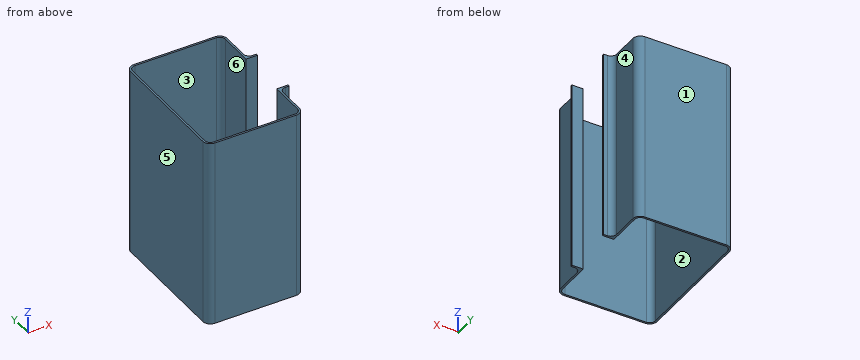
```python
from build123d import *

# Parameters (mm, degrees)
F1_DEPTH = 100


# Not quite as in the source:
# - a feature names something its author has since deleted; it is built from what else it names


with BuildPart() as f1:
    # F0 (on Top) → F1 (new body)
    with BuildSketch(Plane.XY):
        with BuildLine():
            Line((-21.5, 35), (21.5, 35))
            ThreePointArc((21.5, 35), (23.6213203436, 34.1213203436), (24.5, 32))
            Line((24.5, 32), (24.5, 13.625))
            Line((24.5, 13.625), (30.5, 13.625))
            Line((30.5, 13.625), (30.5, 14.625))
            Line((30.5, 14.625), (28.5, 14.625))
            ThreePointArc((28.5, 14.625), (26.3786796564, 15.5036796564), (25.5, 17.625))
            Line((25.5, 17.625), (25.5, 32))
            ThreePointArc((25.5, 32), (24.3284271247, 34.8284271247), (21.5, 36))
            Line((21.5, 36), (-21.5, 36))
            ThreePointArc((-21.5, 36), (-24.3284271247, 34.8284271247), (-25.5, 32))
            Line((-25.5, 32), (-25.5, -32))
            ThreePointArc((-25.5, -32), (-24.3284271247, -34.8284271247), (-21.5, -36))
            Line((-21.5, -36), (21.5, -36))
            ThreePointArc((21.5, -36), (24.3284271247, -34.8284271247), (25.5, -32))
            Line((25.5, -32), (25.5, -17.625))
            ThreePointArc((25.5, -17.625), (26.3786796564, -15.5036796564), (28.5, -14.625))
            Line((28.5, -14.625), (30.5, -14.625))
            Line((30.5, -14.625), (30.5, -13.625))
            Line((30.5, -13.625), (24.5, -13.625))
            Line((24.5, -13.625), (24.5, -32))
            ThreePointArc((24.5, -32), (23.6213203436, -34.1213203436), (21.5, -35))
            Line((21.5, -35), (-21.5, -35))
            ThreePointArc((-21.5, -35), (-23.6213203436, -34.1213203436), (-24.5, -32))
            Line((-24.5, -32), (-24.5, 32))
            ThreePointArc((-24.5, 32), (-23.6213203436, 34.1213203436), (-21.5, 35))
        make_face()
    extrude(amount=F1_DEPTH)


solid = f1.part
```
Geometry: final body of the model. Coordinates: model frame, mm. Face numbers are marked on the shaded views. A direction names the side the tool comes from. Round coordinates to 2 decimals unless told otherwise and drop trailing zeros. Write each loop counter-clockwise with the first axis right and the second up, starting at its lowest first coordinate (ties: lowest second). Pieces come first, ordered by that corner, then holes. Notation, with made-up numbers: M 22.25,-1.75 L 50.25,-1.75 A14 ccw 50.25,7.25 Z; hole C -17,57 d9. An arc over 180 degrees is marked long. Answer in a Markdown table with one row per item. Add a question column.
(1) Draft query along X for the marked faces 1, 2, 3 and 4. Return one class per face: pulls with the +X half, pulls with the -X half, needs draft (parallel to the pull), parting line crosses it, or undercut.
(2) Contact query for flat-ended pins moving along their axis: pin 1 (4.5 mm diameter, centred on y = 26, z = 57.5, fed in from +X); pin 2 (1.5 mm diameter, centred on y = 0.5, z = 78.5, fed in from +X); pin 3 (3 mm diameter, centred on x = 28.5, z = 53, fed in from +Y). Output: stop coordinate, or through.
(3) Cut plane B-B, the plane x = -16.5. Return the cut outline in (y, z), then the cut area to 3 significant figures.
(4) Ray query, L1, parallel to Y at x = 11, z = 9; L2, parallel to X at y = 21.5, z = 56; L3, parallel to X at y = 3.5, z = 18. Return the intervals inside material, ascending.
(5) Cut plane C-C, the plane z = 36. Return the cut outline in (x, y) (3 decimals), then the cut area to 3 significant figures.
(6) Cut plane D-D, the plane y = 0.5. Return the cut outline in (x, z), then the cut area to 3 significant figures.
(7) Cut plane A-A, the plane y = -23. Return the cut outline in (x, z).
(8) Reachability of the marked faces 5 and 6 from +Z, -Z, +X, -X, +Y, -Y: full face, straight path, thin tool, end or side. Return the list, or none.
Established:
| question | item | result |
|---|---|---|
| 1 | face 1 | needs draft |
| 1 | face 2 | undercut |
| 1 | face 3 | undercut |
| 1 | face 4 | pulls with the +X half |
| 2 | pin 1 | x = 25.5 |
| 2 | pin 2 | x = -24.5 |
| 2 | pin 3 | y = 15.03 |
| 3 | outline | M -36,0 L -35,0 L -35,100 L -36,100 Z; M 35,0 L 36,0 L 36,100 L 35,100 Z |
| 3 | area | 200 mm² |
| 4 | L1 | -36 to -35, 35 to 36 |
| 4 | L2 | -25.5 to -24.5, 24.5 to 25.5 |
| 4 | L3 | -25.5 to -24.5 |
| 5 | outline | M -25.5,-32 A4 ccw -21.5,-36 L 21.5,-36 A4 ccw 25.5,-32 L 25.5,-17.625 A3 cw 28.5,-14.625 L 30.5,-14.625 L 30.5,-13.625 L 24.5,-13.625 L 24.5,-32 A3 cw 21.5,-35 L -21.5,-35 A3 cw -24.5,-32 L -24.5,32 A3 cw -21.5,35 L 21.5,35 A3 cw 24.5,32 L 24.5,13.625 L 30.5,13.625 L 30.5,14.625 L 28.5,14.625 A3 cw 25.5,17.625 L 25.5,32 A4 ccw 21.5,36 L -21.5,36 A4 ccw -25.5,32 Z |
| 5 | area | 223 mm² |
| 6 | outline | M -25.5,0 L -24.5,0 L -24.5,100 L -25.5,100 Z |
| 6 | area | 100 mm² |
| 7 | outline | M -25.5,0 L -24.5,0 L -24.5,100 L -25.5,100 Z; M 24.5,0 L 25.5,0 L 25.5,100 L 24.5,100 Z |
| 8 | face 5 | +Z, -Z, -X, +Y, -Y |
| 8 | face 6 | +Z, -Z |
